```python
from build123d import *

# Parameters (mm, degrees)
SKETCH_1_W                  = 60
SKETCH_1_H                  = 76
EXTRUDE_1_DEPTH             = 7.5
SKETCH_2_W                  = 15
SKETCH_2_H                  = 66
CUT_EXTRUDE_2_DEPTH         = 51.68530359
CHAMFER_1_SIZE              = 5
HOLE_WIZARD_6_5_6_5_1_D     = 6.5
HOLE_WIZARD_6_5_6_5_1_DEPTH = 15
HOLE_WIZARD_6_5_6_5_1_TIP   = 1.952797012
SKETCH_6_R                  = 7.5
CUT_EXTRUDE_4_DEPTH         = 51.68530359
SKETCH_7_R                  = 11
CUT_EXTRUDE_5_DEPTH         = 6


with BuildPart() as part:
    # 草图1 → 拉伸1 (new, symmetric)
    with BuildSketch(Plane.XY):
        Rectangle(SKETCH_1_W, SKETCH_1_H)
    extrude(amount=EXTRUDE_1_DEPTH, both=True)

    # 草图2 → 拉伸2 (cut, through all)
    with BuildSketch(Plane.XY.offset(7.5)):
        with Locations((-22.5, 5)):
            Rectangle(SKETCH_2_W, SKETCH_2_H)
        with Locations((22.5, 5)):
            Rectangle(SKETCH_2_W, SKETCH_2_H)
    extrude(amount=-CUT_EXTRUDE_2_DEPTH, mode=Mode.SUBTRACT)

    # 倒角1
    chamfer_1_edges = [part.edges().sort_by_distance(p)[0] for p in [
        (-15, 38, 0),
        (15, 38, 0),
    ]]
    chamfer(chamfer_1_edges, length=CHAMFER_1_SIZE)

    # Ø6.5 (6.5) 直径孔1
    with Locations(Plane.XZ.offset(38)):
        with Locations((-22.5, 0), (22.5, 0)):
            Hole(HOLE_WIZARD_6_5_6_5_1_D / 2, depth=HOLE_WIZARD_6_5_6_5_1_DEPTH)
            with Locations((0, 0, -(HOLE_WIZARD_6_5_6_5_1_DEPTH + HOLE_WIZARD_6_5_6_5_1_TIP / 2))):  # 118° drill point
                Cone(0, HOLE_WIZARD_6_5_6_5_1_D / 2, HOLE_WIZARD_6_5_6_5_1_TIP, mode=Mode.SUBTRACT)

    # 草图6 → 拉伸4 (cut, through all)
    with BuildSketch(Plane.XY.offset(7.5)):
        with Locations((0, 22.5)):
            Circle(SKETCH_6_R)
    extrude(amount=-CUT_EXTRUDE_4_DEPTH, mode=Mode.SUBTRACT)

    # 草图7 → 拉伸5 (cut)
    with BuildSketch(Plane.XY.offset(7.5)):
        with Locations((0, 22.5)):
            Circle(SKETCH_7_R)
    extrude(amount=-CUT_EXTRUDE_5_DEPTH, mode=Mode.SUBTRACT)


solid = part.part
```
Here's how the part is built. I have some questions about the finished solid (model axes, mm). A direction names the side the tool comes from. Round coordinates to 2 decimals unless told otherwise and drop trailing zeros. Loops run counter-clockwise (first coordinate to the right, second up) from the corner with the lowest first, then second, coordinate; pieces in that order, holes last. Notation, with made-up numbers: (-35, -16.75) -> (22, -16.75) arc R18 ccw to (22, -3.75) -> close; hole circle Ø6 at (54, 1). An arc over 180 degrees is marked (long way). Answer as CSV lines item,"result".
1. If we section it at A-A on z = 0: Please give me the cut outline in (x, y), plus the area to 3 significant figures.
Final values:
outline,"(-30, -38) -> (-25.75, -38) -> (-25.75, -28) -> (-30, -28) -> close; (-19.25, -38) -> (19.25, -38) -> (19.25, -28) -> (15, -28) -> (15, 33) -> (10, 38) -> (-10, 38) -> (-15, 33) -> (-15, -28) -> (-19.25, -28) -> close; (25.75, -38) -> (30, -38) -> (30, -28) -> (25.75, -28) -> close; hole circle Ø15 at (0, 22.5)"
area,"2,250 mm^2"
2. Thinking about a two-plate mould opening in X: for faces 1 (the face through (-30, -33, 0)), 2 (the face through (13, 35, 0)), 3 (the face through (-0.976, 29.936, -2.937)), which applies, released by +X, released by -X, zero draft, split by the parting line, or undercut?
Final values:
face 1,"released by -X"
face 2,"released by +X"
face 3,"undercut"
3. If I drill on L1, parallel to Y at x = 0, z = 4.3; L2, parallel to Z at x = -22.5, y = -33; L3, parallel to Y at x = 19.5, z = 3, over which ranges is the centre line in solid material (lowest first)?
Final values:
L1,"y = -38 to 11.5, 33.5 to 38"
L2,"z = -7.5 to -3.25, 3.25 to 7.5"
L3,"y = -38 to -28"
4. If we section it at C-C on y = 22.5: Please give me the cut outline in (x, z).
Final values:
outline,"(-15, -7.5) -> (-7.5, -7.5) -> (-7.5, 1.5) -> (-11, 1.5) -> (-11, 7.5) -> (-15, 7.5) -> close; (7.5, -7.5) -> (15, -7.5) -> (15, 7.5) -> (11, 7.5) -> (11, 1.5) -> (7.5, 1.5) -> close"
5. If we section it at B-B on x = -22.5: Please give me the cut outline in (y, z).
Final values:
outline,"(-38, -7.5) -> (-28, -7.5) -> (-28, -3.25) -> (-38, -3.25) -> close; (-38, 3.25) -> (-28, 3.25) -> (-28, 7.5) -> (-38, 7.5) -> close"
6. If we section it at D-D on z = 4.5: Please give me the cut outline in (x, y), plus the area to 3 significant figures.
Final values:
outline,"(-30, -38) -> (30, -38) -> (30, -28) -> (15, -28) -> (15, 33) -> (10, 38) -> (-10, 38) -> (-15, 33) -> (-15, -28) -> (-30, -28) -> close; hole circle Ø22 at (0, 22.5)"
area,"2,170 mm^2"
7. For pin 1 (1.5 mm diameter, centred on x = 11.5, z = -1, fed in from +Y); pin 2 (8.5 mm diameter, centred on x = -22.5, z = 0, fed in from +Y); pin 3 (4 mm diameter, centred on y = 11, z = -2.5, fed in from -X); pin 4 (6 mm diameter, centred on x = 22.5, z = 0, fed in from +Y), each with a flat end and sliding along its axis, tell me the tip position at first contact or that it passes through.
Final values:
pin 1,"stops at y = 37.25"
pin 2,"stops at y = -28"
pin 3,"stops at x = -15"
pin 4,"passes through"
8. Which directions (+Z, -Z, +X, -X, +Y, -Y) give clear straight access to the entire face, cutting with the end or side of a thin tool? Please do faces 4 (the face through (2, 15, 1.5)), 5 (the face through (-15, 2, 0)), 6 (the face through (15, 2, 0)), 7 (the face through (0, 38, 0)), 8 (the face through (0, -8, -7.5)).
Final values:
face 4,"+Z"
face 5,"+Z, -Z, -X, +Y"
face 6,"+Z, -Z, +X, +Y"
face 7,"+Z, -Z, +X, -X, +Y"
face 8,"-Z, +X, -X, +Y, -Y"
